from build123d import *

# Parameters (mm, degrees)
SKETCH1_R           = 2.5
SKETCH1_R_2         = 1.5
BOSS_EXTRUDE1_DEPTH = 3


with BuildPart() as part:
    # Sketch1 → Boss-Extrude1 (new body)
    with BuildSketch(Plane.XY):
        with BuildLine():
            Line((0.139944022, 3.49720112), (0, 3.5))
            ThreePointArc((0, 3.5), (-3.5, 0), (0, -3.5))
            Line((0, -3.5), (0.139944022, -3.49720112))
            Line((0.139944022, -3.49720112), (50, -2.5))
            ThreePointArc((50, -2.5), (52.5, 0), (50, 2.5))
            Line((50, 2.5), (0.139944022, 3.49720112))
        make_face()
        Circle(SKETCH1_R, mode=Mode.SUBTRACT)
        with Locations((50, 0)):
            Circle(SKETCH1_R_2, mode=Mode.SUBTRACT)
    extrude(amount=BOSS_EXTRUDE1_DEPTH)


solid = part.part
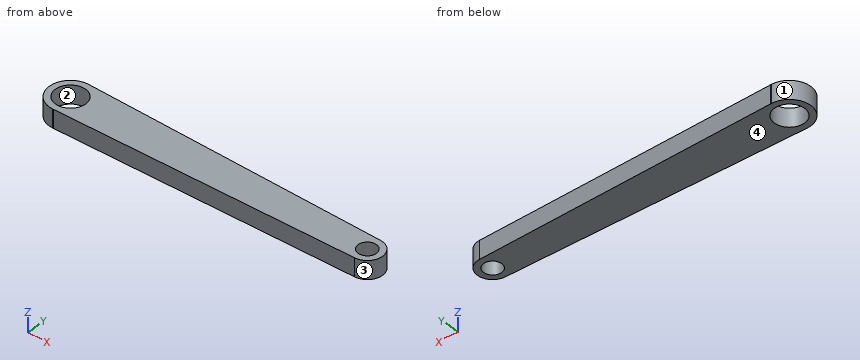
Check sheet for the modelled part. Datum: model origin and axes. Units: mm. Face numbers are marked on the shaded views. Round coordinates to 2 decimals unless told otherwise and drop trailing zeros. Loops run counter-clockwise (first coordinate to the right, second up) from the corner with the lowest first, then second, coordinate; pieces in that order, holes last. Notation, with made-up numbers: (67, 32) - (94, 32) arc R8 cw to (94, 42) - close; hole circle Ø5 at (-33, -10). An arc over 180 degrees is marked (long way). Answer as CSV lines item,"result". Start each with the question number.
Item 1: Release check for a two-part mould opening along X. For the marked faces 1, 2, 3 and 4 record: +X half, -X half, draft (parallel to the pull), parting line (faces both ways), or undercut.
Item 2: Section check A-A (y = 0). Record the boundary of the cut face in (x, z), and give its area (3 significant figures).
Item 3: Depth check by flat-ended pin: P1, Ø2, axis at x = 30.5, y = -0.5, coming from the -Z side. Enter the tip coordinate at first touch or a pass-through.
Item 4: Section check C-C (x = 34.5). Record the boundary of the cut face in (y, z), and give its area (3 significant figures).
Item 5: Section check D-D (x = 17). Record the boundary of the cut face in (y, z), and give its area (3 significant figures).
Item 6: Scan lines: line 1 (Y direction, x = 50, z = 0.6); line 2 (X direction, y = -0.75, z = 1); line 3 (Y direction, x = 49.5, z = 2.95). Record each from-to range of solid material in increasing order. Write a range as [from, to].
Item 7: Section check B-B (z = 1.75). Record the boundary of the cut face in (x, y), and give its area (3 significant figures).
Report:
1,face 1,"-X half"
1,face 2,"undercut"
1,face 3,"+X half"
1,face 4,"draft"
2,outline,"(-3.5, 0) - (-2.5, 0) - (-2.5, 3) - (-3.5, 3) - close; (2.5, 0) - (48.5, 0) - (48.5, 3) - (2.5, 3) - close; (51.5, 0) - (52.5, 0) - (52.5, 3) - (51.5, 3) - close"
2,area,"144 mm2"
3,P1,"stops at z = 0"
4,outline,"(-2.81, 0) - (2.81, 0) - (2.81, 3) - (-2.81, 3) - close"
4,area,"16.9 mm2"
5,outline,"(-3.16, 0) - (3.16, 0) - (3.16, 3) - (-3.16, 3) - close"
5,area,"19.0 mm2"
6,line 1,"y = [-2.5, -1.5], [1.5, 2.5]"
6,line 2,"x = [-3.42, -2.38], [2.38, 48.7], [51.3, 52.38]"
6,line 3,"y = [-2.51, -1.41], [1.41, 2.51]"
7,outline,"(0, -3.5) - (50, -2.5) arc R2.5 ccw to (50, 2.5) - (0, 3.5) arc R3.5 ccw to start; hole circle Ø5 at (0, 0); hole circle Ø3 at (50, 0)"
7,area,"302 mm2"
